from build123d import *
from build123d.topology import SkipClean

# Parameters (mm, degrees)
STOCK_GOUX_START         = -16.954591703
STOCK_GOUX_LIKED_1_DEPTH = 33.909183406
SKETCH1_W                = 5.499999668
SKETCH1_H                = 5.499999668
BOSS_EXTRUDE1_DEPTH      = 33.909183
CUT_EXTRUDE1_DEPTH       = 0.2
SKETCH5_W                = 5.500000112
SKETCH5_H                = 4
CUT_EXTRUDE2_DEPTH       = 116.998760999
CUT_EXTRUDE3_REACH       = 131.039
SKETCH6_R                = 0.64999997
CIRPATTERN1_COUNT        = 2


# Read off the part's stored shape, not the designer's step: Stock-Goux Liked-1
with BuildPart() as part:
    # Stock-Goux Liked-1 outline → Stock-Goux Liked-1 (new body)
    with BuildSketch(Plane(origin=(0, 0, 0), x_dir=(0.7071067811865471, -0.707106781186548, -1.0381022375924514e-12), z_dir=(0.707106781186548, 0.707106781186547, 1.03810223759245e-12)).offset(STOCK_GOUX_START)):
        Polygon((113.704878, -109.20487811), (110.204877888, -109.20487811), (110.204877888, -104.204878204), (109.704877872, -104.204878204), (109.704877872, -109.704877872), (104.204878204, -109.704877872), (104.204878204, -110.204877888), (109.20487811, -110.204877888), (109.20487811, -113.704878), (113.704878, -113.704878), align=None)
    extrude(amount=STOCK_GOUX_LIKED_1_DEPTH)

    # Sketch1 → Boss-Extrude1 (add)
    with SkipClean():  # the faces are left unmerged after this step: merging them gives an invalid solid
        with BuildSketch(Plane(origin=(-11.988706765, -11.988706765, 0), x_dir=(0, 0, 1), z_dir=(-0.7071067811865476, -0.7071067811865476, -1.0381022375924498e-12))):
            with Locations((106.954878038, -106.954878038)):
                Rectangle(SKETCH1_W, SKETCH1_H)
        extrude(amount=-BOSS_EXTRUDE1_DEPTH)

    # Sketch4 → Cut-Extrude1 (cut)
    # profile 1 of 2: a face of its own
    with SkipClean():  # the faces are left unmerged after this step: merging them gives an invalid solid
        with BuildSketch(Plane(origin=(73.683976011, -73.683976011, 109.3690912), x_dir=(-0.577350269189024, -0.5773502691890293, -0.5773502691908239), z_dir=(0.7071067811865546, -0.7071067811865406, -7.406550393246722e-15))):
            Polygon((1.809420407, 5.9526292), (2.820688436, 5.237745386), (-0.821148503, 0.092362774), (-1.331234641, 0.453620787), (1.954432426, 5.095277437), (1.145418003, 5.667693303), align=None)
        # profile 2 of 2: a face of its own
        with BuildSketch(Plane(origin=(73.683976011, -73.683976011, 109.3690912), x_dir=(-0.577350269189024, -0.5773502691890293, -0.5773502691908239), z_dir=(0.7071067811865546, -0.7071067811865406, -7.406550393246722e-15))):
            with BuildLine():
                add(Edge.make_bspline(
                    [(2.877099219, 1.335109376), (2.935838558, 1.417405427), (3.049870438, 1.577168434), (3.226094966, 1.802117563), (3.397935378, 2.009052811), (3.565846799, 2.196717165), (3.731042214, 2.364759935), (3.892218805, 2.513489688), (4.049493585, 2.6446306), (4.206341025, 2.754179531), (4.360025947, 2.849477701), (4.513266986, 2.930884131), (4.665815664, 3.001483938), (4.818515166, 3.0586782), (4.970617605, 3.103726049), (5.122467787, 3.135794894), (5.273974853, 3.1545795), (5.424485375, 3.162398332), (5.57291168, 3.158649601), (5.71885612, 3.143489484), (5.861127958, 3.116280577), (6.000815508, 3.080299839), (6.135189962, 3.029311133), (6.267827501, 2.971265194), (6.395960204, 2.899842577), (6.477761121, 2.844757759), (6.518936158, 2.817030449)],
                    knots=[0, 0, 0, 0, 1.645926604, 3.195270974, 4.650990582, 6.024584171, 7.293755489, 8.485788563, 9.594173223, 10.624575106, 11.597800751, 12.536632912, 13.44787851, 14.332590146, 15.188862484, 16.028272991, 16.856251527, 17.671878837, 18.479816086, 19.271126229, 20.057755364, 20.836377498, 21.616069947, 22.394783881, 23.192003771, 24, 24, 24, 24], degree=3))
                add(Edge.make_bspline(
                    [(6.518936158, 2.817030449), (6.55976619, 2.787194518), (6.640619439, 2.728112222), (6.751575276, 2.627837993), (6.852736041, 2.520826461), (6.947411421, 2.408793466), (7.028861928, 2.287452494), (7.103669209, 2.160876743), (7.168780117, 2.027049302), (7.222899915, 1.885998413), (7.267901579, 1.739512987), (7.300866367, 1.587191132), (7.322801886, 1.429869211), (7.330695863, 1.26694766), (7.330109349, 1.099094482), (7.315823786, 0.925626884), (7.288049754, 0.747536935), (7.251766786, 0.563275675), (7.200579852, 0.372683439), (7.132420302, 0.175939832), (7.049730345, -0.028750132), (6.948143476, -0.239331033), (6.832538734, -0.457983193), (6.701011573, -0.684022575), (6.552211688, -0.916111082), (6.444401149, -1.071082575), (6.389188562, -1.150447515)],
                    knots=[0, 0, 0, 0, 0.816802234, 1.617464211, 2.412328798, 3.195799554, 3.984556322, 4.770779044, 5.57064894, 6.386329449, 7.210029482, 8.044686804, 8.902317584, 9.773878156, 10.678405193, 11.613358687, 12.583410326, 13.589949519, 14.647090142, 15.769568218, 16.952951381, 18.212671993, 19.546052618, 20.949315433, 22.437664922, 24, 24, 24, 24], degree=3))
                add(Edge.make_bspline(
                    [(6.389188562, -1.150447515), (6.332868819, -1.228410619), (6.222953274, -1.380566091), (6.053980888, -1.59680156), (5.886092947, -1.795129872), (5.720527442, -1.977104519), (5.555468389, -2.14060009), (5.392619894, -2.288332456), (5.229879441, -2.416533943), (5.06880285, -2.528231787), (4.908319086, -2.62376275), (4.750132346, -2.708320198), (4.591787049, -2.778366159), (4.43448342, -2.83591584), (4.277857668, -2.882112619), (4.121447774, -2.915750879), (3.965574172, -2.934147856), (3.811266823, -2.942458126), (3.659376547, -2.93720443), (3.510689745, -2.920194702), (3.36547389, -2.894056504), (3.223504099, -2.855347129), (3.084985381, -2.806224594), (2.95051219, -2.744153097), (2.819392507, -2.672081016), (2.735930058, -2.616047292), (2.693926142, -2.587847355)],
                    knots=[0, 0, 0, 0, 1.555964073, 3.036672929, 4.438544486, 5.759244319, 7.015609763, 8.196038705, 9.314565292, 10.364961386, 11.364978532, 12.334676732, 13.26524597, 14.163730662, 15.042916469, 15.905349198, 16.748578791, 17.579666054, 18.403330588, 19.204079274, 19.99928434, 20.788072044, 21.582240779, 22.374243664, 23.181810095, 24, 24, 24, 24], degree=3))
                add(Edge.make_bspline(
                    [(2.693926142, -2.587847355), (2.653972599, -2.558392707), (2.574601729, -2.49987872), (2.465975341, -2.401634599), (2.365605333, -2.297566017), (2.2736202, -2.1872728), (2.192619489, -2.068887343), (2.120885752, -1.944019679), (2.056991419, -1.813489721), (2.003797834, -1.675531189), (1.960019447, -1.532477258), (1.930351112, -1.383658885), (1.908865252, -1.230366615), (1.902666695, -1.072067221), (1.904295565, -0.908849471), (1.920445231, -0.741043703), (1.947114369, -0.568163649), (1.985744352, -0.389662384), (2.037667139, -0.203869884), (2.109148043, -0.010956547), (2.193927603, 0.192170439), (2.298441048, 0.403140358), (2.41709386, 0.624619201), (2.556318665, 0.8530354), (2.707928908, 1.093119466), (2.819610096, 1.252873979), (2.877099219, 1.335109376)],
                    knots=[0, 0, 0, 0, 0.808779551, 1.606704505, 2.384003051, 3.164613963, 3.944979997, 4.719198901, 5.510630197, 6.311633127, 7.127324821, 7.946144414, 8.782972344, 9.648016313, 10.525999108, 11.442197657, 12.393424347, 13.376370558, 14.417965243, 15.535316785, 16.727980085, 18.004753573, 19.371800586, 20.822810559, 22.364506719, 24, 24, 24, 24], degree=3))
            make_face()
            with BuildLine():
                add(Edge.make_bspline(
                    [(3.35665651, 0.981483574), (3.306978299, 0.911008481), (3.210677048, 0.774392459), (3.078907805, 0.570533382), (2.960189865, 0.377340166), (2.855654482, 0.194154463), (2.764740054, 0.020871626), (2.688020563, -0.142683987), (2.626604617, -0.296952862), (2.578871536, -0.44232507), (2.542700408, -0.580836662), (2.517352523, -0.715193163), (2.500264654, -0.845562566), (2.494109389, -0.973145552), (2.496347211, -1.096867933), (2.508033102, -1.217594791), (2.527765974, -1.33483755), (2.568655303, -1.483337821), (2.636042316, -1.657054286), (2.74538605, -1.843427475), (2.878111587, -2.00703341), (2.986845425, -2.092357104), (3.041191767, -2.135002804)],
                    knots=[0, 0, 0, 0, 1.477317626, 2.863781319, 4.158438436, 5.362400069, 6.477048567, 7.510710121, 8.456474969, 9.320360837, 10.130971237, 10.907558897, 11.661836949, 12.382033042, 13.094195176, 13.780270445, 14.458724783, 15.128447747, 16.416912985, 17.638070278, 18.819482119, 20, 20, 20, 20], degree=3))
                add(Edge.make_bspline(
                    [(3.041191767, -2.135002804), (3.099800739, -2.17244124), (3.216225144, -2.246811213), (3.413201595, -2.319023125), (3.622686973, -2.359717176), (3.805834636, -2.366647976), (3.95654946, -2.355929609), (4.071529863, -2.334291982), (4.187465506, -2.305679231), (4.303749507, -2.265403285), (4.421139745, -2.216249685), (4.537600801, -2.154256666), (4.65562294, -2.084375634), (4.732050575, -2.03119598), (4.771159716, -2.003983172)],
                    knots=[0, 0, 0, 0, 1.344638482, 2.671071166, 4.036222541, 5.467361339, 6.209241076, 6.960484297, 7.73186595, 8.521933696, 9.343145882, 10.195949186, 11.076840779, 12, 12, 12, 12], degree=3))
                add(Edge.make_bspline(
                    [(4.771159716, -2.003983172), (4.82003051, -1.9686221), (4.919374766, -1.896740325), (5.060918815, -1.774154816), (5.203980243, -1.643204395), (5.346378414, -1.50118221), (5.486261966, -1.346204267), (5.625768107, -1.181134288), (5.765465845, -1.005346674), (5.854185711, -0.881592057), (5.899454988, -0.818446313)],
                    knots=[0, 0, 0, 0, 0.88015219, 1.789168058, 2.730971114, 3.71133991, 4.723490847, 5.777526881, 6.865983973, 8, 8, 8, 8], degree=3))
                add(Edge.make_bspline(
                    [(5.899454988, -0.818446313), (5.943440103, -0.754631373), (6.029543374, -0.629710132), (6.150227485, -0.443464789), (6.259152206, -0.262044693), (6.355718777, -0.085418135), (6.441234167, 0.086343364), (6.515300272, 0.253071347), (6.577842064, 0.414764781), (6.629318725, 0.571342113), (6.668108931, 0.723318751), (6.699830384, 0.869038513), (6.718294541, 1.009907895), (6.729255617, 1.144940449), (6.729305449, 1.27510735), (6.719388817, 1.399803316), (6.699117623, 1.519074129), (6.658532604, 1.667727811), (6.589724745, 1.839773408), (6.485308774, 2.027436778), (6.35071278, 2.187039301), (6.243987251, 2.272131395), (6.190751062, 2.314576523)],
                    knots=[0, 0, 0, 0, 1.329008706, 2.601607309, 3.804917726, 4.956779838, 6.052592714, 7.094265147, 8.08401922, 9.024445114, 9.918561811, 10.772732897, 11.579936426, 12.352846219, 13.094480438, 13.809401199, 14.495531423, 15.16575916, 16.448433362, 17.663221731, 18.834382256, 20, 20, 20, 20], degree=3))
                add(Edge.make_bspline(
                    [(6.190751062, 2.314576523), (6.132614295, 2.352127809), (6.016155599, 2.427349979), (5.81770787, 2.498184297), (5.606353968, 2.539715843), (5.382213361, 2.546580658), (5.149380752, 2.518724602), (4.913135228, 2.450090337), (4.677174981, 2.338776518), (4.482367978, 2.216674302), (4.323401293, 2.097053878), (4.19971893, 1.986444491), (4.06914087, 1.861579711), (3.934519899, 1.718976231), (3.796468021, 1.558053158), (3.652668391, 1.381505856), (3.505185008, 1.187646731), (3.407224802, 1.051674271), (3.35665651, 0.981483574)],
                    knots=[0, 0, 0, 0, 0.946200866, 1.895415318, 2.86683806, 3.890638819, 4.95642944, 6.069637659, 7.24797886, 8.522380418, 9.215378954, 9.973389102, 10.795730965, 11.692243744, 12.6608267, 13.702269491, 14.813882584, 16, 16, 16, 16], degree=3))
            make_face(mode=Mode.SUBTRACT)
        extrude(amount=CUT_EXTRUDE1_DEPTH, mode=Mode.SUBTRACT)

    # Sketch5 → Cut-Extrude2 (cut, symmetric)
    with BuildSketch(Plane(origin=(77.926616474, -77.926616474, 0), x_dir=(0, 0, -1), z_dir=(0.7071067811865549, -0.7071067811865401, -7.502698527565898e-15))):
        with Locations((-110.954877944, 14.954591703)):
            Rectangle(SKETCH5_W, SKETCH5_H)
    cut_extrude2 = extrude(amount=CUT_EXTRUDE2_DEPTH, both=True, mode=Mode.SUBTRACT)

    # Sketch6 → Cut-Extrude3 (cut, up to next)
    with BuildSketch(Plane.XY.offset(108.204877888), mode=Mode.PRIVATE) as cut_extrude3_sk1:
        with Locations((86.026236134, -64.877249727)):
            Circle(SKETCH6_R)
    cut_extrude3_tool1 = extrude(cut_extrude3_sk1.sketch, amount=-CUT_EXTRUDE3_REACH, mode=Mode.PRIVATE) & part.part
    cut_extrude3 = cut_extrude3_tool1.solids().sort_by_distance((86.026236, -64.87725, 108.204878))[0]
    add(cut_extrude3, mode=Mode.SUBTRACT)

    # CirPattern1: Cut-Extrude2, Cut-Extrude3 ×2 about axis
    cirpattern1_axis = Axis((0, 0, 0), (0.49999999999973677, -0.5000000000002639, 0.7071067811865471))
    add([cut_extrude2.rotate(cirpattern1_axis, i * 360 / CIRPATTERN1_COUNT) for i in range(1, CIRPATTERN1_COUNT)], mode=Mode.SUBTRACT)
    add([cut_extrude3.rotate(cirpattern1_axis, i * 360 / CIRPATTERN1_COUNT) for i in range(1, CIRPATTERN1_COUNT)], mode=Mode.SUBTRACT)


solid = part.part
Verification items for the finished model (mm, model axes). A direction names the side the tool comes from. Coordinates: 2 decimals unless noted, no trailing zeros. Write each loop counter-clockwise with the first axis right and the second up, starting at its lowest first coordinate (ties: lowest second). Pieces come first, ordered by that corner, then holes. Notation, with made-up numbers: M 72,23.25 L 122,23.25 A28 ccw 122,52.25 Z; hole C 38.25,45.25 d11. An arc over 180 degrees is marked long. Use a Markdown table: item, result.
Q1. Go/stop test with flat-tipped pins: P1, Ø6, axis at x = 73, y = -66.5, coming from the -Z side; P2, Ø10, axis at x = 86.5, y = -71.5, coming from the -Z side; P3, Ø5.5, axis at x = 86, y = -65, coming from the +Z side; P4, Ø1.5, axis at x = 78.5, z = 107.5, coming from the -Y side. Record where each tip stops, or that it passes through.
Reply:
| item | result |
|---|---|
| P1 | passes through |
| P2 | stops at z = 104.2 |
| P3 | stops at z = 110.2 |
| P4 | stops at y = -78.1 |
Q2. Sectioned sample at C-C, the plane x = 83.75. Record the boundary of the cut face in (y, z), plus the area to 3 significant figures.
Reply:
| item | result |
|---|---|
| outline | M -77.05,109.2 L -72.1,109.2 L -72.1,104.2 L -63.62,104.2 L -63.62,108.2 L -65.43,108.2 L -65.43,110.2 L -70.69,110.2 L -70.69,113.7 L -77.05,113.7 Z |
| area | 74.5 mm² |
Q3. Set-up check for faces 4 (the face through (79, -79, 109.205)), 5 (the face through (65.958, -87.067, 107.914)), 6 (the face through (74, -77, 110.205)), 7 (the face through (86, -66, 108.205)): record each of +Z, -Z, +X, -X, +Y, -Y from which the full face is reachable in a straight line by a thin tool's end or side.
Reply:
| item | result |
|---|---|
| face 4 | -Z, +X, -Y |
| face 5 | +Z, -Z, -Y |
| face 6 | +Z, -X, +Y |
| face 7 | +Z, +X, +Y |
Q4. Thickness scan on line 1 (Z direction, x = 70.5, y = -77.5); line 2 (Z direction, x = 83.25, y = -64.75); line 3 (X direction, y = -85.5, z = 113). Record the ranges inside material, lowest first.
Reply:
| item | result |
|---|---|
| line 1 | z = 104.2 to 110.2 |
| line 2 | z = 104.2 to 108.2 |
| line 3 | x = 68.94 to 75.3 |
Q5. Draft check along X on faces 1 (the face through (79, -79, 113.705)), 2 (the face through (64.682, -85.554, 107.325)), 3 (the face through (77.09, -77.35, 111.93)). Enter one of: +X half, -X half, draft (parallel to the pull), parting line (faces both ways), or undercut.
Reply:
| item | result |
|---|---|
| face 1 | draft |
| face 2 | undercut |
| face 3 | -X half |
Q6. Sectioned sample at A-A, the plane z = 112. Record the boundary of the cut face in (x, y).
Reply:
| item | result |
|---|---|
| outline | M 68.06,-86.38 L 71.24,-89.56 L 89.56,-71.24 L 86.38,-68.06 Z |
Q7. Sectioned sample at B-B, the plane y = -81.5. Record the boundary of the cut face in (x, z), plus the area to 3 significant figures.
Reply:
| item | result |
|---|---|
| outline | M 65.87,104.2 L 74.35,104.2 L 74.35,109.2 L 79.3,109.2 L 79.3,113.7 L 72.94,113.7 L 72.94,110.2 L 65.87,110.2 Z |
| area | 78.1 mm² |
